```python
from build123d import *

# Parameters (mm, degrees)
SKETCH001_R   = 5
SKETCH003_R   = 5
POCKET_DEPTH  = 39.997504
SKETCH004_R   = 5.5
SKETCH004_R_2 = 3
PAD_DEPTH     = 10


with BuildPart() as part:
    # Sketch → AdditiveLoft section 0
    with BuildSketch(Plane.XY):
        with BuildLine():
            ThreePointArc((-95, 10), (-105, 0), (-95, -10))
            Line((-95, -10), (-75, -10))
            ThreePointArc((-75, -10), (-65, 0), (-75, 10))
            Line((-95, 10), (-75, 10))
        make_face()
    # Sketch001 → AdditiveLoft section 1
    with BuildSketch(Plane.YZ):
        with Locations((0, 35)):
            Circle(SKETCH001_R)
    # Sketch002 → AdditiveLoft section 2
    with BuildSketch(Plane.XY):
        with BuildLine():
            ThreePointArc((75, 10), (65, 0), (75, -10))
            Line((75, -10), (95, -10))
            ThreePointArc((95, -10), (105, 0), (95, 10))
            Line((75, 10), (95, 10))
        make_face()
    loft()

    # Sketch003 (on Face1 of AdditiveLoft) → Pocket (cut, through all)
    with BuildSketch(Plane(origin=(0, 0, 0), x_dir=(1, 0, 0), z_dir=(0, 0, -1))):
        with Locations((-95, 0)):
            Circle(SKETCH003_R)
        with Locations((95, 0)):
            Circle(SKETCH003_R)
    extrude(amount=-POCKET_DEPTH, mode=Mode.SUBTRACT)

    # Sketch004 (on Face8 of Pocket) → Pad (join)
    with BuildSketch(Plane(origin=(0, 0, 0), x_dir=(1, 0, 0), z_dir=(0, 0, -1))):
        with Locations((-95, 0)):
            Circle(SKETCH004_R)
        with Locations((-95, 0)):
            Circle(SKETCH004_R_2, mode=Mode.SUBTRACT)
        with Locations((95, 0)):
            Circle(SKETCH004_R)
        with Locations((95, 0)):
            Circle(SKETCH004_R_2, mode=Mode.SUBTRACT)
    extrude(amount=PAD_DEPTH)


solid = part.part
```
For this review, take the finished solid that the model builds, in its own axes (mm). A direction names the side the tool comes from. Round coordinates to 2 decimals unless told otherwise and drop trailing zeros.
Q1. We need section A-A, the plane y = 0. State how many separate pieces and enclosed holes the cut face has, plus the area to 3 significant figures.
Findings below:
separate pieces: 3
enclosed holes: 0
area: 2,960 mm2
Q2. Insertion check: P1, Ø3, axis at x = -21.5, z = 32, coming from the -Y side; P2, Ø8, axis at x = -97, y = 2.5, coming from the +Z side; P3, Ø2, axis at y = -6.5, z = 2, coming from the +X side; P4, Ø9.5, axis at x = 95, y = 0, coming from the -Z side. Each pin has a flat end and moves straight along its axis. Give the tip position at first contact, or say it passes through.
Findings below:
P1: stops at y = -5.37
P2: stops at z = 7.01
P3: stops at x = 101.42
P4: stops at z = -10
Q3. Wall thickness on line 1 (X direction, y = 0, z = -3.5); line 2 (Y direction, x = 95, z = -6); line 3 (X direction, y = 0, z = 3): over which ranges is each line inside the solid? List them lowest first.
Findings below:
line 1: x = -100.5 to -98, -92 to -89.5, 89.5 to 92, 98 to 100.5
line 2: y = -5.5 to -3, 3 to 5.5
line 3: x = -100.99 to -100, -90 to -61.66, 61.66 to 90, 100 to 100.99
Q4. Machinability: for faces 1 (the cylindrical face through (90, 0, 4)), 2 (the cylindrical face through (92, 0, -5)), 3 (the cylindrical face through (-100.495, -0.242, -4.93)), which of the approach directions +Z, -Z, +X, -X, +Y, -Y give a long, thin tool a straight path to every point of the face, cutting with its end or side? Answer none if there is none.
Findings below:
face 1: +Z
face 2: +Z, -Z
face 3: -Z
Q5. Mouldability with a two-part tool opening along X and no side actions: class faces 4 (the flat face through (-92.6, 2.4, -10)), 5 (the flat face through (85, 0, 0)) as pulls with the +X half, pulls with the -X half, needs draft (parallel to the pull), parting line crosses it, or undercut.
Findings below:
face 4: needs draft
face 5: undercut
